Here's how the part is built. I have some questions about the finished solid (model axes, mm). Face numbers are marked on the shaded views. A direction names the side the tool comes from. Coordinates: 2 decimals unless noted, no trailing zeros. Loops run counter-clockwise (first coordinate to the right, second up) from the corner with the lowest first, then second, coordinate; pieces in that order, holes last. Notation, with made-up numbers: (-18, -37.5) -> (28, -37.5) arc R33 cw to (28, -6.5) -> close; hole circle Ø7 at (-8, 58.5). An arc over 180 degrees is marked (long way). Answer as a JSON object with one key per item and string values. Group by question number.
1) I want a section at B-B (y = 2.25). Write out the boundary of the cut face in (x, z).
2) Which directions (+Z, -Z, +X, -X, +Y, -Y) give clear straight access to the entire face, cutting with the end or side of a thin tool? Please do the marked faces 1 and 2.
3) I want a section at A-A (y = 7). Write out the boundary of the cut face in (x, z).
4) If we mould it in two halves opening along Z, with no side actions, what happens to the marked faces 3, 4 and 5? For each: +Z half, -Z half, draft (parallel to the pull), parting line (faces both ways), or undercut.
5) I need wall thicknesses on probe 1 along Z at (x, y) = (0, 8.75); probe 2 along Z at (x, y) = (0, 6.5). Which ranges of each line are inside material? Lowest first, please. Write a range as [from, to].
6) I want a section at C-C (y = 4.25). Write out the boundary of the cut face in (x, z).
7) I'm going to push flat-ended pins straight in: pin 1 (3.5 mm diameter, centred on x = 0, z = 0, fed in from -Y); pin 2 (1.5 mm diameter, centred on x = 0, z = 0, fed in from +Y); pin 3 (1 mm diameter, centred on x = 1, y = 9, fed in from -Z); pin 4 (0.7 mm diameter, centred on x = 2, y = 7, fed in from +Z). Where does each tip first touch, or does it pass through?
```python
from build123d import *

# Parameters (mm, degrees)
F2_SIZE       = 0.635
F3_R          = 0.254
F5_DEPTH      = 2.54
F5_DEPTH_BACK = 2.54


with BuildPart() as f1:
    # F0 (on Right) → F1 (revolve)
    with BuildSketch(Plane.YZ):
        Polygon((0, 0.3175), (0, 0), (2.54, 0), (2.54, 1.5494), (12.7, 1.5494), (12.7, 3.0988), (1.2192, 3.0988), (1.2192, 0.3175), align=None)
    revolve(axis=Axis((0, 1.27, 0), (0, -1, 0)))

    # F2
    f2_edges = [f1.edges().sort_by_distance(p)[0] for p in [
        (0, 1.2192, -3.0988),
        (0, 12.7, -1.5494),
        (0, 12.7, -3.0988),
    ]]
    chamfer(f2_edges, length=F2_SIZE)

    # F3
    f3_edges = [f1.edges().sort_by_distance(p)[0] for p in [
        (0, 0, -0.3175),
    ]]
    fillet(f3_edges, radius=F3_R)

    # F4 (on Right) → F5 (join, two sides)
    with BuildSketch(Plane.YZ) as f5_sk:
        Polygon((6.35, -2.603163), (6.35, -3.81), (6.8326, -3.81), (7.3152, -2.974112), (7.3152, -2.603163), align=None)
    extrude(amount=F5_DEPTH)
    extrude(f5_sk.sketch, amount=-F5_DEPTH_BACK)


solid = f1.part
```
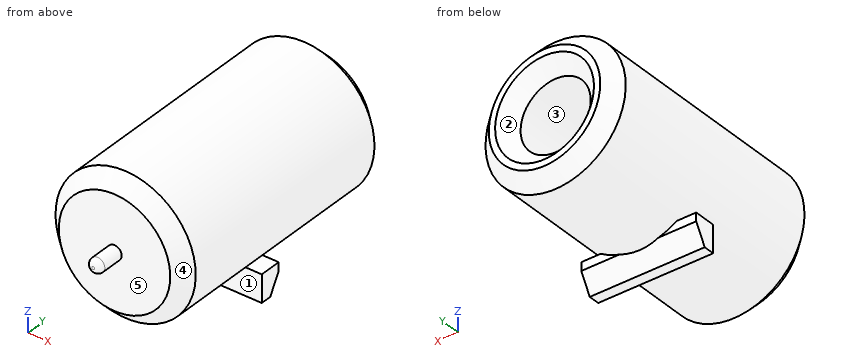
Determined:
{
 "1": {"outline": "circle Ø6.2 at (0, 0)"},
 "2": {"face 1": "-Z, -Y", "face 2": "+Y"},
 "3": {"outline": "(-2.54, -3.52) -> (2.54, -3.52) -> (2.54, -2.6) -> (1.68, -2.6) arc R3.1 ccw (long way) to (-1.68, -2.6) -> (-2.54, -2.6) -> close; hole circle Ø3.1 at (0, 0)"},
 "4": {"face 3": "undercut", "face 4": "parting line", "face 5": "draft"},
 "5": {"probe 1": "[-3.1, -1.55], [1.55, 3.1]", "probe 2": "[-3.81, -1.55], [1.55, 3.1]"},
 "6": {"outline": "circle Ø6.2 at (0, 0); hole circle Ø3.1 at (0, 0)"},
 "7": {"pin 1": "y = 0", "pin 2": "y = 2.54", "pin 3": "z = -3.06", "pin 4": "z = 2.62"}
}
